Work out the finished part from the listing and answer in its coordinate system (mm). Face numbers are marked on the shaded views. Coordinates: 2 decimals unless noted, no trailing zeros. Write each loop counter-clockwise with the first axis right and the second up, starting at its lowest first coordinate (ties: lowest second). Pieces come first, ordered by that corner, then holes. Notation, with made-up numbers: (-39, 25) - (-2, 25) arc R23 ccw to (-2, 38) - close; hole circle Ø5 at (63.5, 39). An arc over 180 degrees is marked (long way). Answer as a JSON object with one key per item and string values. Group by question number.
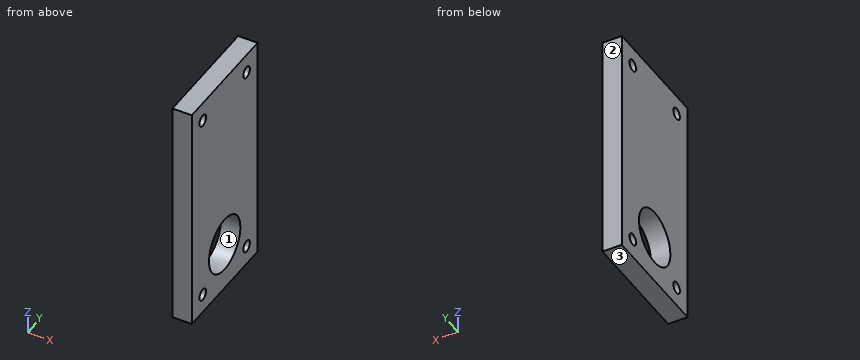
from build123d import *

# Parameters (mm, degrees)
CROQUIS1_W              = 160
CROQUIS1_H              = 60
SALIENTE_EXTRUIR1_DEPTH = 10
CROQUIS2_R              = 14.29
CORTAR_EXTRUIR1_DEPTH   = 87.02325267
CROQUIS3_W              = 40
CROQUIS3_H              = 60
CORTAR_EXTRUIR2_DEPTH   = 87.02325267
CROQUIS4_R              = 3
CORTAR_EXTRUIR3_DEPTH   = 87.02325267


with BuildPart() as part:
    # Croquis1 → Saliente-Extruir1 (new body)
    with BuildSketch(Plane(origin=(0, 0, 0), x_dir=(0, 0, -1), z_dir=(1, 0, 0))):
        Rectangle(CROQUIS1_W, CROQUIS1_H)
    extrude(amount=SALIENTE_EXTRUIR1_DEPTH)

    # Croquis2 → Cortar-Extruir1 (cut, through all)
    with BuildSketch(Plane.ZY):
        with Locations((-58.2308, 0)):
            Circle(CROQUIS2_R)
        with Locations((-15, 0)):
            Circle(CROQUIS2_R)
    extrude(amount=-CORTAR_EXTRUIR1_DEPTH, mode=Mode.SUBTRACT)

    # Croquis3 → Cortar-Extruir2 (cut, through all)
    with BuildSketch(Plane.ZY):
        with Locations((-60, 0)):
            Rectangle(CROQUIS3_W, CROQUIS3_H)
    extrude(amount=-CORTAR_EXTRUIR2_DEPTH, mode=Mode.SUBTRACT)

    # Croquis4 → Cortar-Extruir3 (cut, through all)
    with BuildSketch(Plane.ZY):
        with Locations((70, 20)):
            Circle(CROQUIS4_R)
        with Locations((-30, 20)):
            Circle(CROQUIS4_R)
        with Locations((-30, -20)):
            Circle(CROQUIS4_R)
        with Locations((70, -20)):
            Circle(CROQUIS4_R)
    extrude(amount=-CORTAR_EXTRUIR3_DEPTH, mode=Mode.SUBTRACT)


solid = part.part
Q1. Consider L1, parallel to Y at x = 2, z = 70; L2, parallel to Y at x = 3, z = -32; L3, parallel to Y at x = 2.75, z = -14.5. Determine where each line is inside the solid, lowest interval first. Write a range as from..to.
Q2. Section A-A on z = -15 is taken. Determine the outline of the cut face in (x, y).
Q3. Section D-D on z = 70 is taken. Determine the outline of the cut face in (x, y), plus the area to 3 significant figures.
Q4. Section B-B on y = -20 is taken. Determine the outline of the cut face in (x, z).
Q5. Flat-ended cylindrical pins translate along their axes: pin 1 Ø8 at (y, z) = (20, 70) entering from -X; pin 2 Ø5 at (y, z) = (20, -30) entering from -X. Find the tip coordinate at first contact, or state that the pin passes through.
Q6. For a pull along Y with two mould halves and no side action, classify the marked faces 1, 2 and 3 as +Y half, -Y half, draft (parallel to the pull), parting line (faces both ways), or undercut.
Q7. Section C-C on x = 1.25 is taken. Determine the outline of the cut face in (y, z), plus the area to 3 significant figures.
Numbers:
{
 "1": {"L1": "y = -30..-23, -17..17, 23..30", "L2": "y = -30..-22.24, -17.76..17.76, 22.24..30", "L3": "y = -30..-14.28, 14.28..30"},
 "2": {"outline": "(0, -30) - (10, -30) - (10, -14.29) - (0, -14.29) - close; (0, 14.29) - (10, 14.29) - (10, 30) - (0, 30) - close"},
 "3": {"outline": "(0, -30) - (10, -30) - (10, -23) - (0, -23) - close; (0, -17) - (10, -17) - (10, 17) - (0, 17) - close; (0, 23) - (10, 23) - (10, 30) - (0, 30) - close", "area": "480 mm²"},
 "4": {"outline": "(0, -40) - (10, -40) - (10, -33) - (0, -33) - close; (0, -27) - (10, -27) - (10, 67) - (0, 67) - close; (0, 73) - (10, 73) - (10, 80) - (0, 80) - close"},
 "5": {"pin 1": "stops at x = 0", "pin 2": "passes through"},
 "6": {"face 1": "undercut", "face 2": "+Y half", "face 3": "draft"},
 "7": {"outline": "(-30, -40) - (30, -40) - (30, 80) - (-30, 80) - close; hole circle Ø6 at (-20, -30); hole circle Ø6 at (-20, 70); hole circle Ø28.58 at (0, -15); hole circle Ø6 at (20, -30); hole circle Ø6 at (20, 70)", "area": "6,450 mm²"}
}
